The listing builds one solid part. Answer for the finished solid, in the listing's coordinates (mm). A direction names the side the tool comes from. Round coordinates to 2 decimals unless told otherwise and drop trailing zeros. Loops run counter-clockwise (first coordinate to the right, second up) from the corner with the lowest first, then second, coordinate; pieces in that order, holes last. Notation, with made-up numbers: (-10, -1.75) -> (37, -1.75) arc R13 cw to (37, 7.25) -> close; hole circle Ø9 at (26, -34). An arc over 180 degrees is marked (long way). Use a Markdown table: item, result. Add a question column.
Q1. Which of the six approach directions +Z, -Z, +X, -X, +Y, -Y give full straight-line access (tool end or side, diameter ignored) to faces 1 (the cylindrical face through (-51.99, 7.08, 8.94)), 2 (the cylindrical face through (43.151, 10.354, 8.421)), 3 (the flat face through (-9, 82, 7.435))?
Q2. Section B-B on y = 45.5 is taken. Give the vertices of the cut face in (x, z), then the cut area to 3 significant figures.
Q3. Section C-C on z = 8.1 is taken. Give the number of separate pieces and of enclosed holes in the cut face, then the cut area to 3 significant figures.
Q4. Given pin 1 Ø3 at (x, y) = (-48, 8) entering from +Z; pin 2 Ø4.5 at (x, y) = (24.01, 83.45) entering from +Z; pin 3 Ø12 at (x, y) = (-34, 62.5) entering from -Z, each flat-ended and moving along its own axis, determine where each tip first touches the part or whether it passes through.
Q5. For a pull along Y with two mould halves and no side action, classify faces 4 (the cylindrical face through (-24.145, 6.511, 8.421)), 5 (the flat face through (-1, 8, 9.435)) as released by +Y, released by -Y, zero draft, split by the parting line, or undercut.
Q6. Section A-A on x = -40 is taken. Give the vertices of the cut face in (y, z), then the cut area to 3 significant figures.
Q7. Consider line 1 (X direction, y = 31.5, z = 8.35); line 2 (Y direction, x = -11, z = 8.8); line 3 (X direction, y = 50, z = 8.45). Determine where each line is inside the solid, lowest interval first.
from build123d import *

# Parameters (mm, degrees)
SKETCH1_W                  = 109.5
SKETCH1_H                  = 83
BOSS_EXTRUDE1_DEPTH        = 2
F_3_2_3_2_DIAMETER_HOLE1_D = 3.2
F_2_7_2_7_DIAMETER_HOLE1_D = 2.7
SKETCH12_R                 = 3
CUT_EXTRUDE1_DEPTH         = 1
FILLET1_R                  = 3
FILLET2_R                  = 1


with BuildPart() as part:
    # Sketch1 → Boss-Extrude1 (new body)
    with BuildSketch(Plane.XY.offset(7.43465612)):
        with Locations((-0.743641502, 44.95185693)):
            Rectangle(SKETCH1_W, SKETCH1_H)
        with BuildLine():
            Line((-42.493641502, 80.45185693), (41.006358498, 80.45185693))
            ThreePointArc((41.006358498, 80.45185693), (43.127678842, 79.573177274), (44.006358498, 77.45185693))
            Line((44.006358498, 77.45185693), (44.006358498, 54.95185693))
            Line((44.006358498, 54.95185693), (48.006358498, 54.95185693))
            Line((48.006358498, 54.95185693), (48.006358498, 44.95185693))
            Line((48.006358498, 44.95185693), (48.006358498, 34.95185693))
            Line((48.006358498, 34.95185693), (44.006358498, 34.95185693))
            Line((44.006358498, 34.95185693), (44.006358498, 12.45185693))
            ThreePointArc((44.006358498, 12.45185693), (43.127678842, 10.330536587), (41.006358498, 9.45185693))
            Line((41.006358498, 9.45185693), (-42.493641502, 9.45185693))
            ThreePointArc((-42.493641502, 9.45185693), (-44.614961845, 10.330536587), (-45.493641502, 12.45185693))
            Line((-45.493641502, 12.45185693), (-45.493641502, 77.45185693))
            ThreePointArc((-45.493641502, 77.45185693), (-44.614961845, 79.573177274), (-42.493641502, 80.45185693))
        make_face(mode=Mode.SUBTRACT)
    extrude(amount=BOSS_EXTRUDE1_DEPTH)

    # Ø3.2 (3.2) Diameter Hole1 (through all)
    with Locations(Plane.XY.offset(9.43465612)):
        with Locations((-48.993641502, 6.95185693), (-48.993641502, 82.95185693), (47.506358498, 82.95185693), (47.506358498, 6.95185693)):
            Hole(F_3_2_3_2_DIAMETER_HOLE1_D / 2)

    # Ø2.7 (2.7) Diameter Hole1 (through all)
    with Locations(Plane(origin=(-25.493641502, 83.45185693, 9.43465612), x_dir=(1, 0, 0), z_dir=(0, 0, 1))):
        with Locations((0, 0), (49.5, 0), (49.5, -77), (0, -77)):
            Hole(F_2_7_2_7_DIAMETER_HOLE1_D / 2)

    # Sketch12 → Cut-Extrude1 (cut)
    with BuildSketch(Plane.XY.offset(9.43465612)):
        with Locations((-48.993641502, 82.95185693)):
            Circle(SKETCH12_R)
        with Locations((47.506358498, 82.95185693)):
            Circle(SKETCH12_R)
        with Locations((47.506358498, 6.95185693)):
            Circle(SKETCH12_R)
        with Locations((-48.993641502, 6.95185693)):
            Circle(SKETCH12_R)
    extrude(amount=-CUT_EXTRUDE1_DEPTH, mode=Mode.SUBTRACT)

    # Fillet1
    fillet1_edges = [part.edges().sort_by_distance(p)[0] for p in [
        (48.006358498, 34.95185693, 8.43465612),
        (48.006358498, 54.95185693, 8.43465612),
    ]]
    fillet(fillet1_edges, radius=FILLET1_R)

    # Fillet2
    fillet2_edges = [part.edges().sort_by_distance(p)[0] for p in [
        (44.006358498, 34.95185693, 8.43465612),
        (44.006358498, 54.95185693, 8.43465612),
    ]]
    fillet(fillet2_edges, radius=FILLET2_R - 0.0001)  # a hair under: the kernel refuses the full size


solid = part.part
Checked values:
| question | item | result |
|---|---|---|
| 1 | face 1 | +Z |
| 1 | face 2 | +Z, -Z |
| 1 | face 3 | -Z, +X, -X, +Y, -Y |
| 2 | outline | (-55.49, 7.43) -> (-45.49, 7.43) -> (-45.49, 9.43) -> (-55.49, 9.43) -> close; (48.01, 7.43) -> (54.01, 7.43) -> (54.01, 9.43) -> (48.01, 9.43) -> close |
| 2 | area | 32.0 mm2 |
| 3 | separate pieces | 1 |
| 3 | enclosed holes | 9 |
| 3 | area | 2,610 mm2 |
| 4 | pin 1 | stops at z = 8.43 |
| 4 | pin 2 | stops at z = 9.43 |
| 4 | pin 3 | passes through |
| 5 | face 4 | undercut |
| 5 | face 5 | zero draft |
| 6 | outline | (3.45, 7.43) -> (9.45, 7.43) -> (9.45, 9.43) -> (3.45, 9.43) -> close; (80.45, 7.43) -> (86.45, 7.43) -> (86.45, 9.43) -> (80.45, 9.43) -> close |
| 6 | area | 24.0 mm2 |
| 7 | line 1 | x = -55.49 to -45.49, 44.01 to 54.01 |
| 7 | line 2 | y = 3.45 to 9.45, 80.45 to 86.45 |
| 7 | line 3 | x = -55.49 to -45.49, 48.01 to 54.01 |
